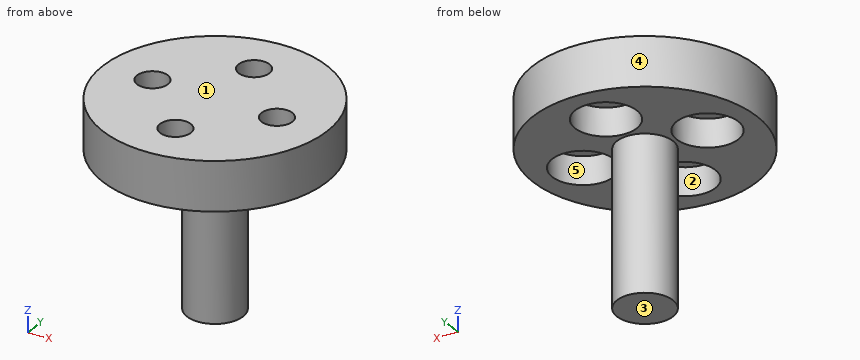
from build123d import *

# Parameters (mm, degrees)
CBORE_FOR_M2_SHCS2_D           = 2.2
CBORE_FOR_M2_SHCS2_CBORE_D     = 4.4
CBORE_FOR_M2_SHCS2_CBORE_DEPTH = 2


with BuildPart() as part:
    # Sketch1 → Revolve1 (revolve)
    with BuildSketch(Plane(origin=(0, 0, 0), x_dir=(1, 0, 0), z_dir=(0, 1, 0))):
        Polygon((0, 0), (8, 0), (8, 3.5), (2, 3.5), (2, 14.5), (0, 14.5), align=None)
    revolve(axis=Axis((0, 0, -14.5), (0, 0, 1)))

    # CBORE for M2 SHCS2 (through all)
    with Locations(Plane(origin=(0, 0, -3.5), x_dir=(-1, 0, 0), z_dir=(0, 0, -1))):
        with Locations((4.49122807, 0), (0.023889511, 4.49122807), (-4.467338559, -0.023889511), (0, -4.515117581)):
            CounterBoreHole(CBORE_FOR_M2_SHCS2_D / 2, CBORE_FOR_M2_SHCS2_CBORE_D / 2, CBORE_FOR_M2_SHCS2_CBORE_DEPTH)


solid = part.part
Geometry check sheet. Reference: the model listing, model coordinates, mm. Face numbers are marked on the shaded views. A direction names the side the tool comes from. Give positions to 0.01 mm unless a question says otherwise; leave off trailing zeros. Write each loop counter-clockwise with the first axis right and the second up, starting at its lowest first coordinate (ties: lowest second). Pieces come first, ordered by that corner, then holes. Notation, with made-up numbers: (-6.5, 28.5) - (43.5, 28.5) arc R25 ccw to (43.5, 58.5) - close; hole circle Ø9 at (-14, 75). An arc over 180 degrees is marked (long way). Put each result on its own line as item: value.
1. Sectioned sample at D-D, the plane y = 4.75. Enter the section's corners in (x, z), plus the area to 3 significant figures.
Ans:
outline: (-6.44, -3.5) - (-2.21, -3.5) - (-2.21, -1.5) - (-1.09, -1.5) - (-1.09, 0) - (-6.44, 0) - close; (1.05, -1.5) - (2.16, -1.5) - (2.16, -3.5) - (6.44, -3.5) - (6.44, 0) - (1.05, 0) - close
area: 33.1 mm²
2. Sectioned sample at C-C, the plane z = -5. Enter the section's corners in (x, y), plus the area to 3 significant figures.
Ans:
outline: circle Ø4 at (0, 0)
area: 12.6 mm²
3. Thickness scan on line 1 (Z direction, x = -4.75, y = 2.75); line 2 (Z direction, x = 1.25, y = -4.25); line 3 (Y direction, x = 2, z = -2.5). Record the ranges inside material, lowest first.
Ans:
line 1: z = -3.5 to 0
line 2: z = -1.5 to 0
line 3: y = -7.75 to -5.43, -3.6 to 3.63, 5.35 to 7.75
4. Go/stop test with flat-tipped pins: pin 1 (3 mm diameter, centred on x = 0, z = -11, fed in from -Y); pin 2 (8 mm diameter, centred on x = 4.5, z = -9, fed in from +Y); pin 3 (2 mm diameter, centred on x = 0, y = 5.5, fed in from -Z). Record where each tip stops, or that it passes through.
Ans:
pin 1: stops at y = -2
pin 2: stops at y = 1.94
pin 3: stops at z = -1.5
5. Set-up check for the marked faces 1 and 2: record each of +Z, -Z, +X, -X, +Y, -Y from which the full face is reachable in a straight line by a thin tool's end or side.
Ans:
face 1: +Z, +X, -X, +Y, -Y
face 2: -Z
6. Draft check along Y on the marked faces 3, 4 and 5. Enter one of: +Y half, -Y half, draft (parallel to the pull), parting line (faces both ways), or undercut.
Ans:
face 3: draft
face 4: parting line
face 5: undercut
7. Sectioned sample at B-B, the plane x = 0. Enter the section's corners in (y, z).
Ans:
outline: (-8, -3.5) - (-6.72, -3.5) - (-6.72, -1.5) - (-5.62, -1.5) - (-5.62, 0) - (-8, 0) - close; (-3.42, -1.5) - (-2.32, -1.5) - (-2.32, -3.5) - (-2, -3.5) - (-2, -14.5) - (2, -14.5) - (2, -3.5) - (2.29, -3.5) - (2.29, -1.5) - (3.39, -1.5) - (3.39, 0) - (-3.42, 0) - close; (5.59, -1.5) - (6.69, -1.5) - (6.69, -3.5) - (8, -3.5) - (8, 0) - (5.59, 0) - close
8. Sectioned sample at A-A, the plane y = 0.5. Enter the section's corners in (x, z), plus the area to 3 significant figures.
Ans:
outline: (-7.98, -3.5) - (-6.63, -3.5) - (-6.63, -1.5) - (-5.47, -1.5) - (-5.47, 0) - (-7.98, 0) - close; (-3.51, -1.5) - (-2.35, -1.5) - (-2.35, -3.5) - (-1.94, -3.5) - (-1.94, -14.5) - (1.94, -14.5) - (1.94, -3.5) - (2.33, -3.5) - (2.33, -1.5) - (3.5, -1.5) - (3.5, 0) - (-3.51, 0) - close; (5.43, -1.5) - (6.6, -1.5) - (6.6, -3.5) - (7.98, -3.5) - (7.98, 0) - (5.43, 0) - close
area: 75.5 mm²
